from build123d import *

# Parameters (mm, degrees)
SKETCH3_W           = 20
SKETCH3_H           = 10
CUT_EXTRUDE1_DEPTH  = 20
SKETCH4_R           = 2.6
CUT_EXTRUDE2_DEPTH  = 26
SKETCH7_R           = 2.6
CUT_EXTRUDE4_DEPTH  = 26
SKETCH8_W           = 16
SKETCH8_H           = 20
CUT_EXTRUDE9_DEPTH  = 15
SKETCH6_W           = 16
SKETCH6_H           = 20
CUT_EXTRUDE10_DEPTH = 15


with BuildPart() as part:
    # Sketch2 → Revolve1 (revolve)
    with BuildSketch(Plane.XY):
        with BuildLine():
            Line((-30, 0), (0, 0))
            Line((0, 0), (0, 30))
            ThreePointArc((0, 30), (-21.213203436, 21.213203436), (-30, 0))
        make_face()
    revolve(axis=Axis((0, 0, 0), (0, 1, 0)))

    # Sketch3 → Cut-Extrude1 (cut)
    with BuildSketch(Plane.XZ):
        Rectangle(SKETCH3_W, SKETCH3_H)
    extrude(amount=-CUT_EXTRUDE1_DEPTH, mode=Mode.SUBTRACT)

    # Sketch4 → Cut-Extrude2 (cut, through all)
    with BuildSketch(Plane(origin=(0, 0, 5), x_dir=(-1, 0, 0), z_dir=(0, 0, -1))):
        with Locations((0, 15)):
            Circle(SKETCH4_R)
        with Locations((0, 5.050125629)):
            Circle(SKETCH4_R)
    extrude(amount=-CUT_EXTRUDE2_DEPTH, mode=Mode.SUBTRACT)

    # Sketch7 → Cut-Extrude4 (cut, through all)
    with BuildSketch(Plane.XY.offset(-5)):
        with Locations((0, 5)):
            Circle(SKETCH7_R)
        with Locations((0, 15)):
            Circle(SKETCH7_R)
    extrude(amount=-CUT_EXTRUDE4_DEPTH, mode=Mode.SUBTRACT)

    # Sketch8 → Cut-Extrude9 (cut)
    with BuildSketch(Plane.XY.offset(-30)):
        with Locations((0, 10)):
            Rectangle(SKETCH8_W, SKETCH8_H)
    extrude(amount=CUT_EXTRUDE9_DEPTH, mode=Mode.SUBTRACT)

    # Sketch6 → Cut-Extrude10 (cut)
    with BuildSketch(Plane.XY.offset(30)):
        with Locations((0, 10)):
            Rectangle(SKETCH6_W, SKETCH6_H)
    extrude(amount=-CUT_EXTRUDE10_DEPTH, mode=Mode.SUBTRACT)


solid = part.part
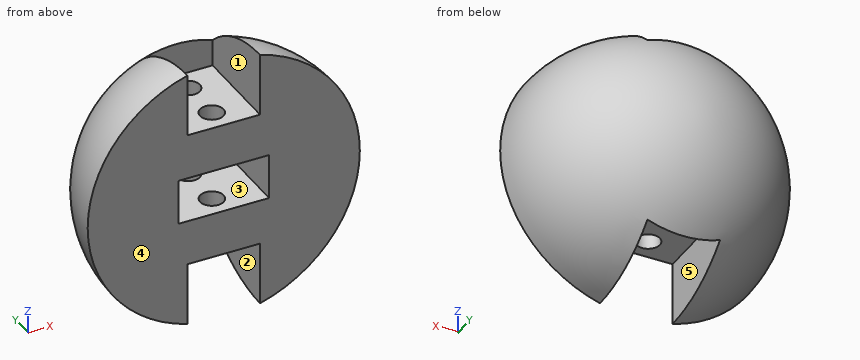
Here's how the part is built. I have some questions about the finished solid (model axes, mm). Face numbers are marked on the shaded views. A direction names the side the tool comes from. Give positions to 0.01 mm unless a question says otherwise; leave off trailing zeros. Loops run counter-clockwise (first coordinate to the right, second up) from the corner with the lowest first, then second, coordinate; pieces in that order, holes last. Notation, with made-up numbers: (26.5, -13) -> (58.5, -13) arc R25 ccw to (58.5, 4) -> close; hole circle Ø7 at (60, 12.5). An arc over 180 degrees is marked (long way). One line per item, written item: value.
Q1. On a 3-axis mill with a long thin cutter (end or side, diameter ignored), from which of +Z, -Z, +X, -X, +Y, -Y can I reach the whole of each face in a straight line? I mean the marked faces 1, 2 and 3. Say none if no direction works.
Answers follow:
face 1: +Z, -Y
face 2: -Z, -Y
face 3: -Y
Q2. Suppose I cut it at C-C on y = 11. Please give me the cut outline in (x, z), then the cut area to 3 significant figures.
Answers follow:
outline: (-8, -26.74) -> (-8, -15) -> (8, -15) -> (8, -26.74) arc R27.91 ccw to (8, 26.74) -> (8, 15) -> (-8, 15) -> (-8, 26.74) arc R27.91 ccw to start; hole (-10, -5) -> (10, -5) -> (10, 5) -> (-10, 5) -> close
area: 1,850 mm^2
Q3. If I drill on line 1 along Y through (x, z) = (0, -7.25); line 2 along Y through (x, z) = (0, 8); line 3 along Z through (x, y) = (-7, 17.5), over which ranges is the centre line in solid material (lowest first)?
Answers follow:
line 1: 0 to 2.4, 7.6 to 12.4, 17.6 to 29.11
line 2: 0 to 2.45, 7.65 to 12.4, 17.6 to 28.91
line 3: -15 to -5, 5 to 15
Q4. Suppose I cut it at B-B on y = 15. Please give me the cut outline in (x, z), then the cut area to 3 significant figures.
Answers follow:
outline: (-10, -5) -> (-10, 5) -> (-2.6, 5) -> (-2.6, 15) -> (-8, 15) -> (-8, 24.72) arc R25.98 ccw to (-8, -24.72) -> (-8, -15) -> (-2.6, -15) -> (-2.6, -5) -> close; (2.6, -15) -> (8, -15) -> (8, -24.72) arc R25.98 ccw to (8, 24.72) -> (8, 15) -> (2.6, 15) -> (2.6, 5) -> (10, 5) -> (10, -5) -> (2.6, -5) -> close
area: 1,480 mm^2
Q5. I'm going to push flat-ended pins straight in: pin 1 Ø11 at (y, z) = (8, 21.5) entering from +X; pin 2 Ø5 at (x, y) = (-19, 17) entering from +Z; pin 3 Ø11 at (y, z) = (13.5, 20) entering from -X; pin 4 Ø4.5 at (x, y) = (0, 5) entering from -Z. Where does each tip first touch, or does it pass through?
Answers follow:
pin 1: x = 24.41
pin 2: z = 19.27
pin 3: x = -23.51
pin 4: through
Q6. We'd pull the mould along X, two halves only. Please class the marked faces 4 and 5: pulls with the +X half, pulls with the -X half, needs draft (parallel to the pull), parting line crosses it, or undercut.
Answers follow:
face 4: needs draft
face 5: undercut
Q7. Suppose I cut it at D-D on z = -24.5. Please give me the cut outline in (x, y).
Answers follow:
outline: (-17.31, 0) -> (-8, 0) -> (-8, 15.35) arc R17.31 ccw to start; (8, 0) -> (17.31, 0) arc R17.31 ccw to (8, 15.35) -> close
Q8. Suppose I cut it at A-A on x = 0. Please give me the cut outline in (y, z).
Answers follow:
outline: (0, -15) -> (2.4, -15) -> (2.4, -5) -> (0, -5) -> close; (0, 5) -> (2.45, 5) -> (2.45, 15) -> (0, 15) -> close; (7.6, -15) -> (12.4, -15) -> (12.4, -5) -> (7.6, -5) -> close; (7.65, 5) -> (12.4, 5) -> (12.4, 15) -> (7.65, 15) -> close; (17.6, -15) -> (20, -15) -> (20, -22.36) arc R30 ccw to (20, 22.36) -> (20, 15) -> (17.6, 15) -> (17.6, 5) -> (20, 5) -> (20, -5) -> (17.6, -5) -> close
